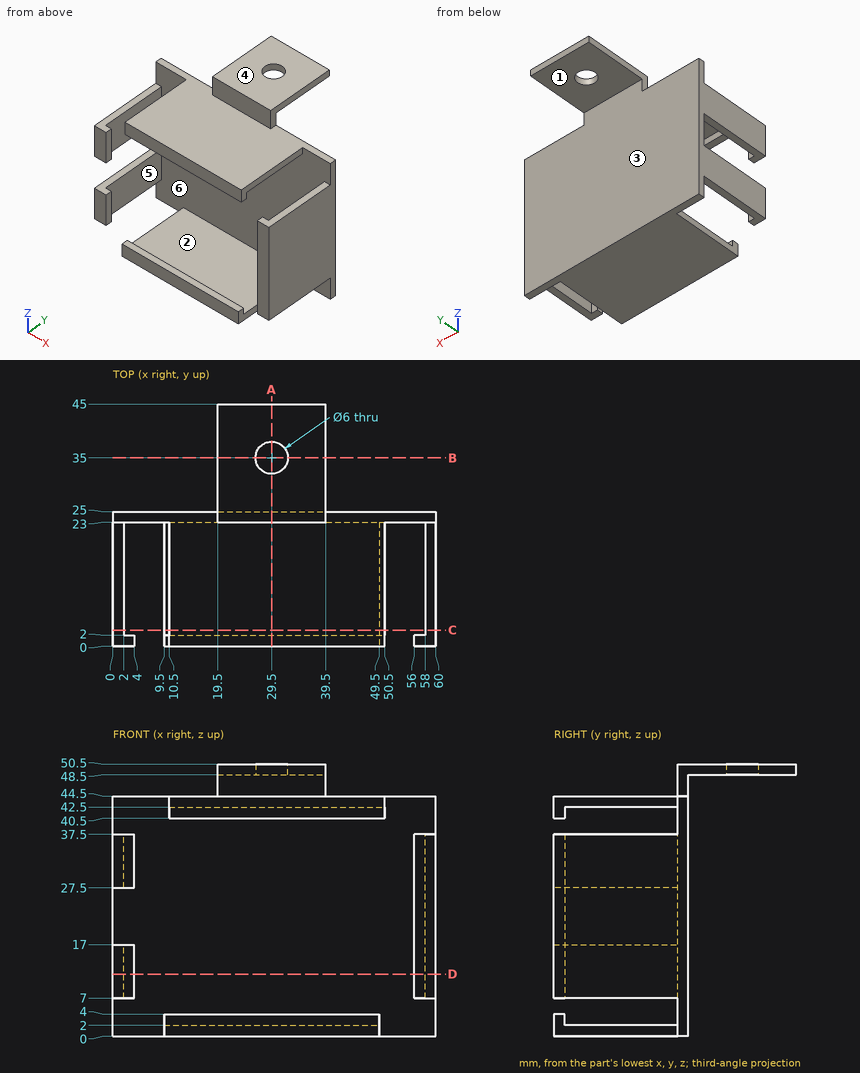
Geometry check sheet. Reference: drawing and pictorial views, mm from the part's lowest x, y, z. A direction names the side the tool comes from. Give positions to 0.01 mm unless a question says otherwise; leave off trailing zeros. Order: outer loops, then holes, each group sorted by start corner. A loop starts at its lowest first (then second) coordinate and runs counter-clockwise, first axis right, second up. Notation, with made-up numbers: M 33.5,22 L 53.5,22 A30 ccw 53.5,61 Z; hole C -8.75,22.5 d8. An arc over 180 degrees is marked long. Answer as a JSON object with one key per item and string values. Group by question number.
1) Cross-section at B-B (y = 35). Enter the section's corners in (x, z).
2) Mould release check, pull along Y, two halves, no side actions. Record for the marked faces 1, 2 and 3: released by +Y, released by -Y, zero draft, split by the parting line, or undercut.
3) Cross-section at C-C (y = 3). Enter the section's corners in (x, z).
4) Access from +Z, -Z, +X, -X, +Y, -Y to the whole of each face (thin tool, end or side, straight path). Record for the marked faces 4, 5 and 6.
5) Cross-section at D-D (z = 11.5). Enter the section's corners in (x, y).
6) Scan lines: line 1 along Z through (x, y) = (16.5, 11.5); line 2 along X through (y, z) = (35, 49.55); line 3 along Y through (x, z) = (29.5, 49.3). Record each from-to range of solid material in increasing order. Write a range as [from, to].
7) Cross-section at A-A (x = 29.5). Enter the section's corners in (y, z), then the cut area to 3 significant figures.
8) Depth check by flat-ended pin: pin 1 Ø1.2 at (y, z) = (9, 42.5) entering from +X; pin 2 Ø3 at (x, y) = (2.5, 15) entering from -Z; pin 3 Ø4 at (x, y) = (44.5, 9.5) entering from +Z; pin 4 Ø1.2 at (x, y) = (3, 14.5) entering from +Z. Enter the tip coordinate at first touch or a pass-through.
Result sheet:
{
 "1": {"outline": "M 19.5,48.5 L 26.5,48.5 L 26.5,50.5 L 19.5,50.5 Z; M 32.5,48.5 L 39.5,48.5 L 39.5,50.5 L 32.5,50.5 Z"},
 "2": {"face 1": "zero draft", "face 2": "undercut", "face 3": "released by +Y"},
 "3": {"outline": "M 0,7 L 2,7 L 2,17 L 0,17 Z; M 0,27.5 L 2,27.5 L 2,37.5 L 0,37.5 Z; M 9.5,0 L 49.5,0 L 49.5,2 L 9.5,2 Z; M 10.5,42.5 L 50.5,42.5 L 50.5,44.5 L 10.5,44.5 Z; M 58,7 L 60,7 L 60,37.5 L 58,37.5 Z"},
 "4": {"face 4": "+Z, +X, -X, +Y, -Y", "face 5": "+Z, -Z", "face 6": "none"},
 "5": {"outline": "M 0,0 L 4,0 L 4,2 L 2,2 L 2,23 L 58,23 L 58,2 L 56,2 L 56,0 L 60,0 L 60,25 L 0,25 Z"},
 "6": {"line 1": "z = [0, 2], [42.5, 44.5]", "line 2": "x = [19.5, 26.5], [32.5, 39.5]", "line 3": "y = [23, 32], [38, 45]"},
 "7": {"outline": "M 0,0 L 25,0 L 25,48.5 L 32,48.5 L 32,50.5 L 23,50.5 L 23,44.5 L 0,44.5 L 0,40.5 L 2,40.5 L 2,42.5 L 23,42.5 L 23,2 L 2,2 L 2,4 L 0,4 Z; M 38,48.5 L 45,48.5 L 45,50.5 L 38,50.5 Z", "area": "229 mm2"},
 "8": {"pin 1": "stops at x = 50.5", "pin 2": "stops at z = 7", "pin 3": "stops at z = 44.5", "pin 4": "passes through"}
}
